Build history of the part. All positions in model axes, mm. Face numbers are marked on the shaded views. A direction names the side the tool comes from. Give positions to 0.01 mm unless a question says otherwise; leave off trailing zeros. Write each loop counter-clockwise with the first axis right and the second up, starting at its lowest first coordinate (ties: lowest second). Pieces come first, ordered by that corner, then holes.
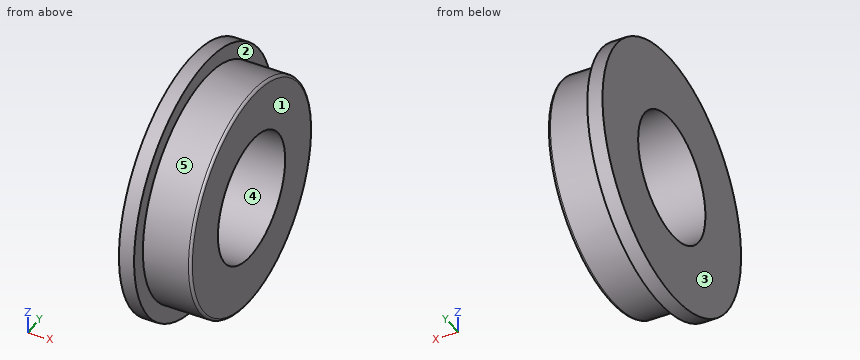
from build123d import *

# Parameters (mm, degrees)
SKETCH1_R           = 5.15
BOSS_EXTRUDE1_DEPTH = 0.6
SKETCH2_R           = 4.5
BOSS_EXTRUDE2_DEPTH = 1.9
SKETCH3_R           = 2.5
CUT_EXTRUDE1_DEPTH  = 8.700324668
FILLET1_R           = 0.1


with BuildPart() as part:
    # Sketch1 → Boss-Extrude1 (new body)
    with BuildSketch(Plane(origin=(0, 0, 0), x_dir=(0, 0, -1), z_dir=(1, 0, 0))):
        Circle(SKETCH1_R)
    extrude(amount=BOSS_EXTRUDE1_DEPTH)

    # Sketch2 → Boss-Extrude2 (add)
    with BuildSketch(Plane(origin=(0.6, 0, 0), x_dir=(0, 0, -1), z_dir=(1, 0, 0))):
        with Locations(Location((0, 0, 0), (0, 0, 180))):
            Circle(SKETCH2_R)
    extrude(amount=BOSS_EXTRUDE2_DEPTH)

    # Sketch3 → Cut-Extrude1 (cut, through all)
    with BuildSketch(Plane(origin=(2.5, 0, 0), x_dir=(0, 0, -1), z_dir=(1, 0, 0))):
        Circle(SKETCH3_R)
    extrude(amount=-CUT_EXTRUDE1_DEPTH, mode=Mode.SUBTRACT)

    # Fillet1
    fillet1_edges = [part.edges().sort_by_distance(p)[0] for p in [
        (2.5, 0, -4.5),
    ]]
    fillet(fillet1_edges, radius=FILLET1_R)


solid = part.part
(1) Mould opens along Y. For the marked faces 3, 4 and 5 say: +Y half, -Y half, draft (parallel to the pull), parting line (faces both ways), or undercut.
(2) Saw through at A-A, the plane y = 0. List the corners of the cut face in (x, z).
(3) 3-axis set-ups, long thin cutter, end or side, ignore diameter. For the marked faces 1 and 2: which of +Z, -Z, +X, -X, +Y, -Y reach the whole face in a straight line?
(4) Probe line 1 (Y direction, x = 0.8, z = 0); line 2 (Z direction, x = 1.7, y = -2.25); line 3 (Y direction, x = 0.5, z = -2.25). List the from-to ranges inside material, lowest first.
(5) Saw through at D-D, the plane x = 1.15. List the corners of the cut face in (y, z), plus the area to 3 significant figures.
(6) Saw through at C-C, the plane x = 0.2. List the corners of the cut face in (y, z), plus the area to 3 significant figures.
Computed values:
1. face 3: draft
1. face 4: undercut
1. face 5: parting line
2. outline: (0, -5.15) - (0.6, -5.15) - (0.6, -4.5) - (2.4, -4.5) arc R0.1 ccw to (2.5, -4.4) - (2.5, -2.5) - (0, -2.5) - close; (0, 2.5) - (2.5, 2.5) - (2.5, 4.4) arc R0.1 ccw to (2.4, 4.5) - (0.6, 4.5) - (0.6, 5.15) - (0, 5.15) - close
3. face 1: +Z, -Z, +X, +Y, -Y
3. face 2: +X
4. line 1: y = -4.5 to -2.5, 2.5 to 4.5
4. line 2: z = -3.9 to -1.09, 1.09 to 3.9
4. line 3: y = -4.63 to -1.09, 1.09 to 4.63
5. outline: circle Ø9 at (0, 0); hole circle Ø5 at (0, 0)
5. area: 44.0 mm2
6. outline: circle Ø10.3 at (0, 0); hole circle Ø5 at (0, 0)
6. area: 63.7 mm2
